Job drawing, mm, ordinate dimensions from the low corner. One solid piece. Round coordinates to 2 decimals unless told otherwise and drop trailing zeros. Loops run counter-clockwise (first coordinate to the right, second up) from the corner with the lowest first, then second, coordinate; pieces in that order, holes last. Notation, with made-up numbers: M 89.25,-30 L 114.25,-30 A28 cw 114.25,9 Z; hole C 68.25,-18.5 d1. An arc over 180 degrees is marked long. Use a Markdown table: item, result. Add a question column.
(1) Wall check: L1, parallel to X at y = 4, z = 100 (3 decimals); L2, parallel to Z at x = 192, y = 7.75. Give the ranges that are in metal, low to high.
(2) Band-saw the part on B-B, the plane x = 85.5. Write the cut outline in (y, z).
(3) Band-saw the part on D-D, the plane z = 12. Write the cut outline in (x, y), and give its area (3 significant figures).
(4) Band-saw the part on A-A, the plane z = 66. Write the cut outline in (x, y).
(5) Band-saw the part on C-C, the plane x = 188. Write the cut outline in (y, z), and give its area (3 significant figures).
(6) Flat gauge pins, fed straight in: P1, Ø1.5, axis at x = 134, y = 4, coming from the -Z side; P2, Ø2.5, axis at x = 100, z = 193.125, coming from the +Y side. Where does each tip first touch, or does it go through?
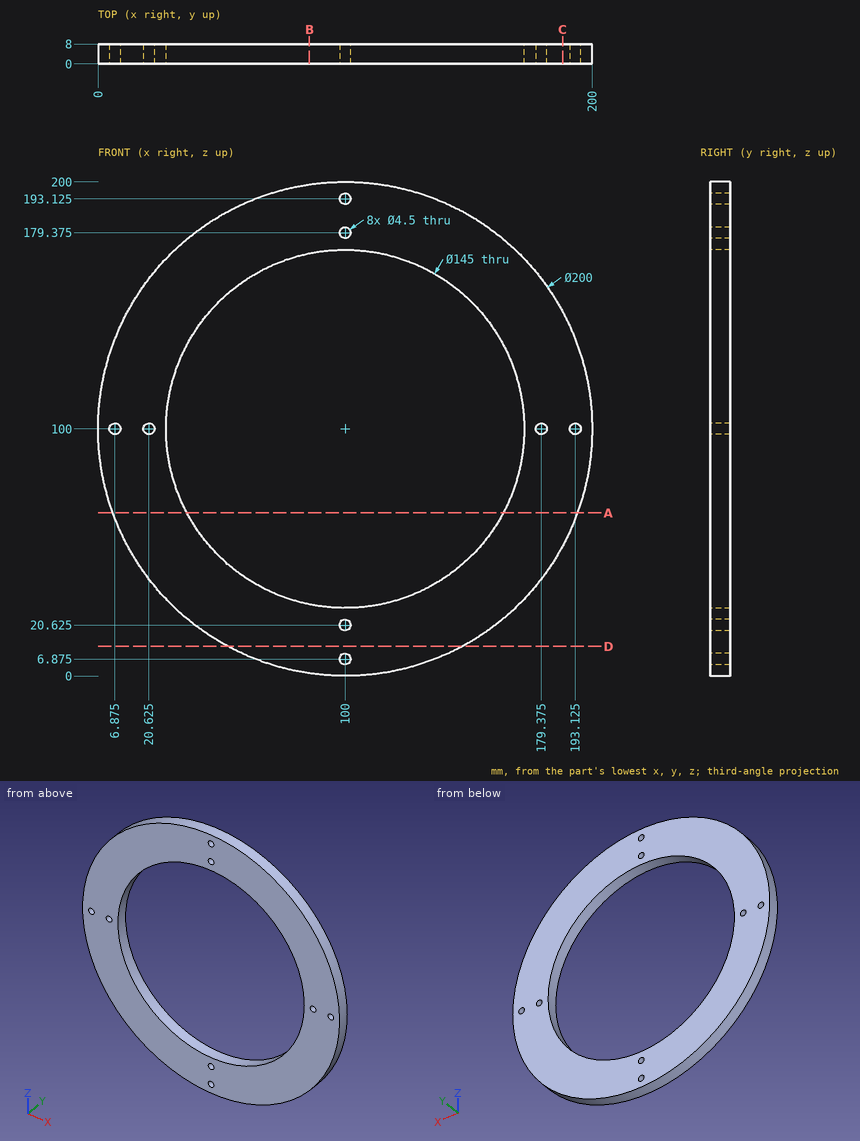
Return value:
| question | item | result |
|---|---|---|
| 1 | L1 | 0 to 4.625, 9.125 to 18.375, 22.875 to 27.5, 172.5 to 177.125, 181.625 to 190.875, 195.375 to 200 |
| 1 | L2 | 60.81 to 98.05, 101.95 to 139.19 |
| 2 | outline | M 0,1.06 L 8,1.06 L 8,28.96 L 0,28.96 Z; M 0,171.04 L 8,171.04 L 8,198.94 L 0,198.94 Z |
| 3 | outline | M 52.5,0 L 147.5,0 L 147.5,8 L 52.5,8 Z |
| 3 | area | 760 mm^2 |
| 4 | outline | M 5.96,0 L 35.97,0 L 35.97,8 L 5.96,8 Z; M 164.03,0 L 194.04,0 L 194.04,8 L 164.03,8 Z |
| 5 | outline | M 0,52.5 L 8,52.5 L 8,147.5 L 0,147.5 Z |
| 5 | area | 760 mm^2 |
| 6 | P1 | z = 5.69 |
| 6 | P2 | through |
